Input: part model. Units: mm. Frame: model coordinates. Face numbers are marked on the shaded views. Give positions to 0.01 mm unless a question says otherwise; leave off trailing zeros. Loops run counter-clockwise (first coordinate to the right, second up) from the corner with the lowest first, then second, coordinate; pieces in that order, holes last. Notation, with made-up numbers: (42, 75) - (55, 75) arc R19 cw to (55, 106) - close; hole circle Ø8 at (6, 36.25). An arc over 180 degrees is marked (long way). Answer as a JSON object with one key per item and string values. Group by question number.
(1) Pin query (flat end, axial travel): P1, Ø2.5, axis at x = 0, z = 0, coming from the -Y side; P2, Ø0.6, axis at x = 0, y = -3, coming from the +Z side; P3, Ø3, axis at y = 4, z = -3.5, coming from the -X side. Return the tip coordinate at first contact, or that it passes through.
(2) Material intervals for L1, parallel to X at y = 2.85, z = 0; L2, parallel to Y at x = 1.75, z = -1.25; L3, parallel to Y at x = -3, z = -1.5, sorted ascending.
(3) Section query B-B (x = 0). Return loops of the section in (y, z), plus the area to 3 significant figures.
(4) Section query C-C (y = 2.5). Return loops of the section in (x, z), plus the area to 3 significant figures.
(5) Section query D-D (z = 0). Return loops of the section in (x, y).
(6) Section query A-A (y = -1). Return loops of the section in (x, z).
(7) Mould query, pull axis Z, two halves, no side actions, for the marked faces 1, 2 and 3. Classes: +Z half, -Z half, draft (parallel to the pull), parting line (faces both ways), or undercut.
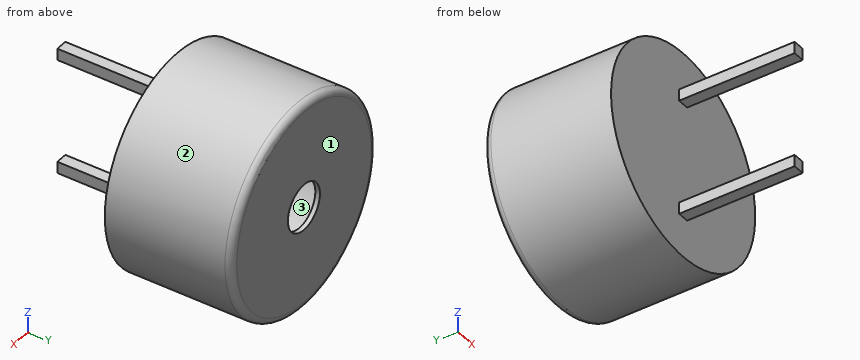
```python
from build123d import *

# Parameters (mm, degrees)
CROQUIS1_R              = 4.5
SALIENTE_EXTRUIR1_DEPTH = 1
CROQUIS2_R              = 4.5
CROQUIS2_R_2            = 3.5
SALIENTE_EXTRUIR2_DEPTH = 4.5
CROQUIS3_R              = 2.296416316
SALIENTE_EXTRUIR3_DEPTH = 2
SALIENTE_EXTRUIR4_START = -0.2
CROQUIS4_R              = 4.5
CROQUIS4_R_2            = 1
SALIENTE_EXTRUIR4_DEPTH = 0.2
CROQUIS5_W              = 0.5
CROQUIS5_H              = 0.5
SALIENTE_EXTRUIR5_DEPTH = 5
REDONDEO1_R             = 0.3


with BuildPart() as part:
    # Croquis1 → Saliente-Extruir1 (new body)
    with BuildSketch(Plane(origin=(0, 0, 0), x_dir=(1, 0, 0), z_dir=(0, 1, 0))):
        with Locations(Location((0, 0, 0), (0, 0, 270))):
            Circle(CROQUIS1_R)
    extrude(amount=SALIENTE_EXTRUIR1_DEPTH)

    # Croquis2 → Saliente-Extruir2 (add)
    with BuildSketch(Plane(origin=(0, 1, 0), x_dir=(1, 0, 0), z_dir=(0, 1, 0))):
        with Locations(Location((0, 0, 0), (0, 0, 270))):
            Circle(CROQUIS2_R)
        with Locations(Location((0, 0, 0), (0, 0, 270))):
            Circle(CROQUIS2_R_2, mode=Mode.SUBTRACT)
    extrude(amount=SALIENTE_EXTRUIR2_DEPTH)

    # Croquis3 → Saliente-Extruir3 (add)
    with BuildSketch(Plane(origin=(0, 1, 0), x_dir=(1, 0, 0), z_dir=(0, 1, 0))):
        with Locations(Location((0, 0, 0), (0, 0, 270))):
            Circle(CROQUIS3_R)
    extrude(amount=SALIENTE_EXTRUIR3_DEPTH)

    # Croquis4 → Saliente-Extruir4 (add)
    with BuildSketch(Plane(origin=(0, 5.5, 0), x_dir=(1, 0, 0), z_dir=(0, 1, 0)).offset(SALIENTE_EXTRUIR4_START)):
        with Locations(Location((0, 0, 0), (0, 0, 270))):
            Circle(CROQUIS4_R)
        with Locations(Location((0, 0, 0), (0, 0, 270))):
            Circle(CROQUIS4_R_2, mode=Mode.SUBTRACT)
    extrude(amount=SALIENTE_EXTRUIR4_DEPTH)

    # Croquis5 → Saliente-Extruir5 (add)
    with BuildSketch(Plane.XZ):
        with Locations((0, -2.5)):
            Rectangle(CROQUIS5_W, CROQUIS5_H)
        with Locations((0, 2.5)):
            Rectangle(CROQUIS5_W, CROQUIS5_H)
    extrude(amount=SALIENTE_EXTRUIR5_DEPTH)

    # Redondeo1
    redondeo1_edges = [part.edges().sort_by_distance(p)[0] for p in [
        (0, 5.5, -4.5),
    ]]
    fillet(redondeo1_edges, radius=REDONDEO1_R)


solid = part.part
```
Recorded:
{
 "1": {"P1": "stops at y = 0", "P2": "stops at z = 2.75", "P3": "stops at x = -4.03"},
 "2": {"L1": "x = -4.5 to -3.5, -2.3 to 2.3, 3.5 to 4.5", "L2": "y = 0 to 3, 5.3 to 5.5", "L3": "y = 0 to 1, 5.3 to 5.5"},
 "3": {"outline": "(-5, -2.75) - (0, -2.75) - (0, -4.5) - (5.2, -4.5) arc R0.3 ccw to (5.5, -4.2) - (5.5, -1) - (5.3, -1) - (5.3, -3.5) - (1, -3.5) - (1, -2.3) - (3, -2.3) - (3, 2.3) - (1, 2.3) - (1, 3.5) - (5.3, 3.5) - (5.3, 1) - (5.5, 1) - (5.5, 4.2) arc R0.3 ccw to (5.2, 4.5) - (0, 4.5) - (0, 2.75) - (-5, 2.75) - (-5, 2.25) - (0, 2.25) - (0, -2.25) - (-5, -2.25) - close", "area": "33.1 mm^2"},
 "4": {"outline": "circle Ø9 at (0, 0); circle Ø4.59 at (0, 0); hole circle Ø7 at (0, 0)", "area": "41.7 mm^2"},
 "5": {"outline": "(-4.5, 0) - (4.5, 0) - (4.5, 5.2) arc R0.3 ccw to (4.2, 5.5) - (1, 5.5) - (1, 5.3) - (3.5, 5.3) - (3.5, 1) - (2.3, 1) - (2.3, 3) - (-2.3, 3) - (-2.3, 1) - (-3.5, 1) - (-3.5, 5.3) - (-1, 5.3) - (-1, 5.5) - (-4.2, 5.5) arc R0.3 ccw to (-4.5, 5.2) - close"},
 "6": {"outline": "(-0.25, -2.75) - (0.25, -2.75) - (0.25, -2.25) - (-0.25, -2.25) - close; (-0.25, 2.25) - (0.25, 2.25) - (0.25, 2.75) - (-0.25, 2.75) - close"},
 "7": {"face 1": "draft", "face 2": "parting line", "face 3": "undercut"}
}
